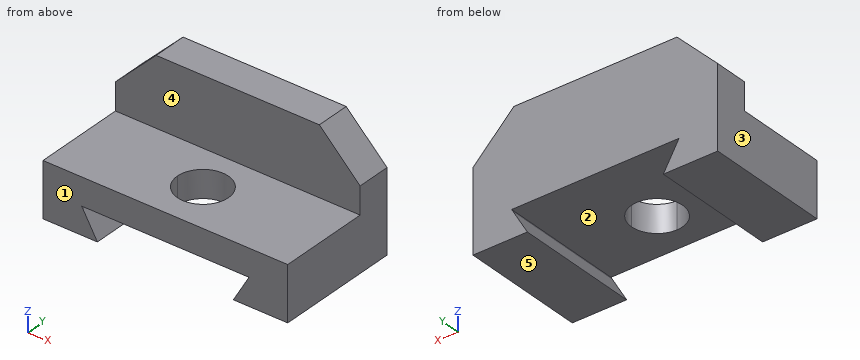
from build123d import *

# Parameters (mm, degrees)
F0_W     = 19.05
F0_H     = 15.875
F0_W_2   = 76.2
F1_DEPTH = 57.15
F2_DEPTH = 25.4
F4_DEPTH = 15.875
F6_DEPTH = 58.7502


with BuildPart() as f1:
    # F0 (on Top) → F1 (new body)
    with BuildSketch(Plane.XY):
        with Locations((-47.625, 28.5877)):
            Rectangle(F0_W, F0_H)
        with Locations((0, 28.5877)):
            Rectangle(F0_W_2, F0_H)
        with Locations((47.625, 28.5877)):
            Rectangle(F0_W, F0_H)
    extrude(amount=F1_DEPTH)

    # F0 (on Top) → F2 (join)
    with BuildSketch(Plane.XY):
        with BuildLine():
            ThreePointArc((-11.90625, 0), (0, 11.90625), (11.90625, 0))
            Line((11.90625, 0), (57.15, 0))
            Line((57.15, 0), (57.15, 20.6502))
            Line((57.15, 20.6502), (38.1, 20.6502))
            Line((38.1, 20.6502), (-38.1, 20.6502))
            Line((-38.1, 20.6502), (-57.15, 20.6502))
            Line((-57.15, 20.6502), (-57.15, 0))
            Line((-57.15, 0), (-11.90625, 0))
        make_face()
        with BuildLine():
            ThreePointArc((0, -11.90625), (-8.41899, -8.41899), (-11.90625, 0))
            Line((-11.90625, 0), (-57.15, 0))
            Line((-57.15, 0), (-57.15, -22.225))
            Line((-57.15, -22.225), (0, -22.225))
            Line((0, -22.225), (0, -11.90625))
        make_face()
        with BuildLine():
            Line((57.15, 0), (11.90625, 0))
            ThreePointArc((11.90625, 0), (8.41899, -8.41899), (0, -11.90625))
            Line((0, -11.90625), (0, -22.225))
            Line((0, -22.225), (57.15, -22.225))
            Line((57.15, -22.225), (57.15, 0))
        make_face()
    extrude(amount=F2_DEPTH)

    # F3 (on face) → F4 (cut)
    with BuildSketch(Plane.XZ.offset(-20.6502)):
        Polygon((-38.1, 57.15), (-57.15, 57.15), (-57.15, 38.1), align=None)
        Polygon((57.15, 57.15), (38.1, 57.15), (57.15, 38.1), align=None)
    extrude(amount=-F4_DEPTH, mode=Mode.SUBTRACT)

    # F5 (on face) → F6 (cut)
    with BuildSketch(Plane.XZ.offset(22.225)):
        Polygon((-38.550498, 11.778808), (-31.75, 0), (0, 0), (0, 12.7), (-39.082348, 12.7), align=None)
        Polygon((0, 12.7), (0, 0), (31.75, 0), (38.550498, 11.778808), (39.082348, 12.7), align=None)
    extrude(amount=-F6_DEPTH, mode=Mode.SUBTRACT)


solid = f1.part
Could you check a few things on this model? Use its own coordinates, in mm. Face numbers are marked on the shaded views. A direction names the side the tool comes from. Give positions to 0.01 mm unless a question says otherwise; leave off trailing zeros. Write each loop counter-clockwise with the first axis right and the second up, starting at its lowest first coordinate (ties: lowest second). Pieces come first, ordered by that corner, then holes. Notation, with made-up numbers: (26.25, 6.5) - (40.25, 6.5) arc R29 ccw to (40.25, 44.5) - close; hole circle Ø6 at (-27, 15.25). An arc over 180 degrees is marked (long way). Use CSV: the item, a comma, the result in double quotes. Start each with the question number.
Item 1: If I drill on line 1 along Y through (x, z) = (34, 29); line 2 along Z through (x, y) = (28, 33); line 3 along Z through (x, y) = (13.5, 10), over which ranges is the centre line in solid material (lowest first)?
Item 2: I'm going to push flat-ended pins straight in: pin 1 (10 mm diameter, centred on x = -37, z = 43.5, fed in from -Y); pin 2 (13 mm diameter, centred on x = 28.5, y = 0.5, fed in from +Z). Where does each tip first touch, or does it pass through?
Item 3: If we mould it in two halves opening along X, with no side actions, what happens to the marked faces 1, 2 and 3? For each: pulls with the +X half, pulls with the -X half, needs draft (parallel to the pull), parting line crosses it, or undercut.
Item 4: I want a section at C-C, the plane z = 9.5. Please give me the cut outline in (x, y) (3 decimals), then the cut area to 3 significant figures.
Item 5: I want a section at A-A, the plane y = 9.5. Please give me the cut outline in (x, z).
Item 6: I want a section at B-B, the plane x = 16. Please give me the cut outline in (y, z) (3 decimals), then the cut area to 3 significant figures.
Item 7: For the marked faces 4 and 5, which set-ups out of +Z, -Z, +X, -X, +Y, -Y let a thin tool reach every point of the face, with its end or its side?
Item 8: I want a section at D-D, the plane y = -5.5. Please give me the cut outline in (x, z).
Findings:
1,line 1,"y = 20.65 to 36.53"
1,line 2,"z = 12.7 to 57.15"
1,line 3,"z = 12.7 to 25.4"
2,pin 1,"stops at y = 20.65"
2,pin 2,"stops at z = 25.4"
3,face 1,"needs draft"
3,face 2,"undercut"
3,face 3,"pulls with the -X half"
4,outline,"(-57.15, -22.225) - (-37.235, -22.225) - (-37.235, 36.525) - (-57.15, 36.525) - close; (37.235, -22.225) - (57.15, -22.225) - (57.15, 36.525) - (37.235, 36.525) - close"
4,area,"2,340 mm2"
5,outline,"(-57.15, 0) - (-31.75, 0) - (-38.55, 11.78) - (-39.08, 12.7) - (-7.18, 12.7) - (-7.18, 25.4) - (-57.15, 25.4) - close; (7.18, 12.7) - (39.08, 12.7) - (38.55, 11.78) - (31.75, 0) - (57.15, 0) - (57.15, 25.4) - (7.18, 25.4) - close"
6,outline,"(-22.225, 12.7) - (36.525, 12.7) - (36.525, 57.15) - (20.65, 57.15) - (20.65, 25.4) - (-22.225, 25.4) - close"
6,area,"1,250 mm2"
7,face 4,"+Z, +X, -X, -Y"
7,face 5,"-Z, +X, -X, +Y, -Y"
8,outline,"(-57.15, 0) - (-31.75, 0) - (-38.55, 11.78) - (-39.08, 12.7) - (-10.56, 12.7) - (-10.56, 25.4) - (-57.15, 25.4) - close; (10.56, 12.7) - (39.08, 12.7) - (38.55, 11.78) - (31.75, 0) - (57.15, 0) - (57.15, 25.4) - (10.56, 25.4) - close"
